Check sheet for the drawn part. Datum: minimum x, y, z corner. Units: mm. A direction names the side the tool comes from. Round coordinates to 2 decimals unless told otherwise and drop trailing zeros. Order: outer loops, then holes, each group sorted by start corner. A loop starts at its lowest first (then second) coordinate and runs counter-clockwise, first axis right, second up.
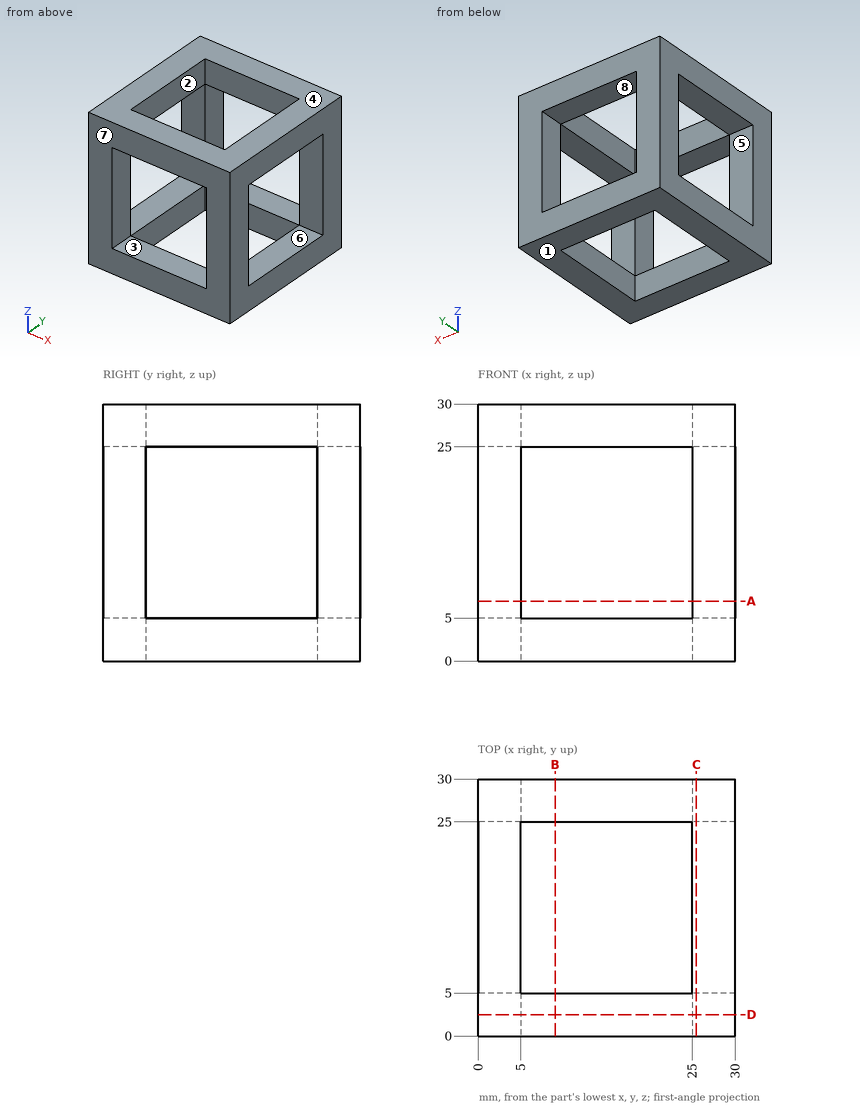
(1) Sectioned sample at A-A, the plane z = 7. Record the cut outline in (x, y).
Returned:
outline: (0, 0) - (5, 0) - (5, 5) - (0, 5) - close; (0, 25) - (5, 25) - (5, 30) - (0, 30) - close; (25, 0) - (30, 0) - (30, 5) - (25, 5) - close; (25, 25) - (30, 25) - (30, 30) - (25, 30) - close
(2) Material ranges on line 1 (Z direction, x = 10.5, y = 4.75), recorded low to high.
Returned:
line 1: z = 0 to 5, 25 to 30
(3) Draft check along Y on the marked faces 6, 7 and 8. Enter one of: released by +Y, released by -Y, zero draft, split by the parting line, or undercut.
Returned:
face 6: undercut
face 7: released by -Y
face 8: zero draft
(4) Set-up check for the marked faces 1, 2, 3, 4 and 5: record each of +Z, -Z, +X, -X, +Y, -Y from which the full face is reachable in a straight line by a thin tool's end or side.
Returned:
face 1: -Z, +X, -X, +Y, -Y
face 2: +Z, -Z
face 3: +Y, -Y
face 4: +Z, +X, -X, +Y, -Y
face 5: +X, -X
(5) Sectioned sample at C-C, the plane x = 25.5. Record the cut outline in (y, z).
Returned:
outline: (0, 0) - (30, 0) - (30, 30) - (0, 30) - close; hole (5, 5) - (25, 5) - (25, 25) - (5, 25) - close
